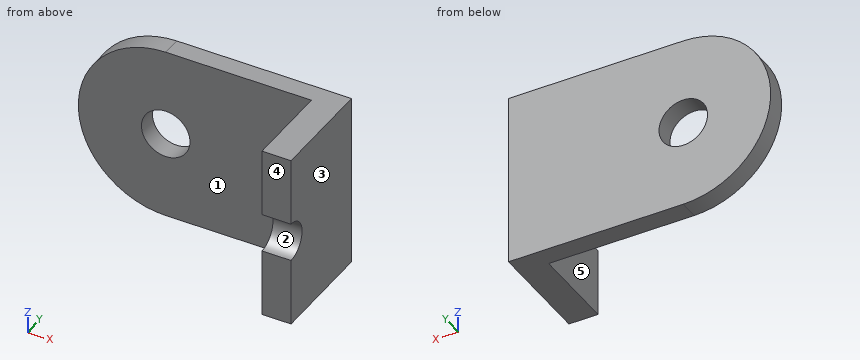
from build123d import *

# Parameters (mm, degrees)
SKETCH1_R           = 2.5
BOSS_EXTRUDE1_DEPTH = 2
BOSS_EXTRUDE2_DEPTH = 3


with BuildPart() as part:
    # Sketch1 → Boss-Extrude1 (new body)
    with BuildSketch(Plane(origin=(0, 0, 0), x_dir=(1, 0, 0), z_dir=(0, 1, 0))):
        with BuildLine():
            Line((0, 9), (18, 9))
            Line((18, 9), (18, -9))
            Line((18, -9), (0, -9))
            ThreePointArc((0, -9), (-9, 0), (0, 9))
        make_face()
        with Locations(Location((0, 0, 0), (0, 0, 270))):
            Circle(SKETCH1_R, mode=Mode.SUBTRACT)
    extrude(amount=BOSS_EXTRUDE1_DEPTH)

    # Sketch2 → Boss-Extrude2 (add)
    with BuildSketch(Plane(origin=(18, 0, 0), x_dir=(0, 0, -1), z_dir=(1, 0, 0))):
        with BuildLine():
            Line((9, 0), (-9, 0))
            Line((-9, 0), (-9, -9))
            Line((-9, -9), (-2, -9))
            ThreePointArc((-2, -9), (0, -7), (2, -9))
            Line((2, -9), (9, -9))
            Line((9, -9), (9, 0))
        make_face()
    extrude(amount=-BOSS_EXTRUDE2_DEPTH)


solid = part.part
Design review of the part built by this model. Coordinates are the model's own, in mm. Face numbers are marked on the shaded views. A direction names the side the tool comes from. Coordinates: 2 decimals unless noted, no trailing zeros. Loops run counter-clockwise (first coordinate to the right, second up) from the corner with the lowest first, then second, coordinate; pieces in that order, holes last. Notation, with made-up numbers: (25, 58) -> (34, 58) arc R7 ccw to (34, 70) -> close; hole circle Ø2 at (37.5, -8.75). An arc over 180 degrees is marked (long way). Use a Markdown table: item, result. Add a question column.
Item 1: Machinability: for the marked faces 1 and 2, which of the approach directions +Z, -Z, +X, -X, +Y, -Y give a long, thin tool a straight path to every point of the face, cutting with its end or side? Answer none if there is none.
Item 2: Clearance check with a flat-ended pin moving along its axis: P1, Ø5.5, axis at x = -1.5, z = -4.5, coming from the -Y side. State where the tip first meets the part, or that it passes through.
Item 3: We need section A-A, the plane z = 0. Write out the cut boundary in (x, y), and give its area (3 significant figures).
Item 4: We need section C-C, the plane x = 16. Write out the cut boundary in (y, z).
Item 5: Wall thickness on L1, parallel to X at y = 1.55, z = 0; L2, parallel to X at y = -0.75, z = 3.25; L3, parallel to Y at x = 9.25, z = 5.5: over which ranges is each line inside the solid? List them lowest first. Write a range as from..to.
Item 6: The part is to be moulded in two halves that separate along X. For the marked faces 3, 4 and 5, say which applies: +X half, -X half, draft (parallel to the pull), parting line (faces both ways), or undercut.
Item 7: We need section D-D, the plane z = -3.75. Write out the cut boundary in (x, y), and give its area (3 significant figures).
Item 8: We need section B-B, the plane y = -7.5. Write out the cut boundary in (x, z), and give its area (3 significant figures).
Numbers:
| question | item | result |
|---|---|---|
| 1 | face 1 | +Z, -Z, -X, -Y |
| 1 | face 2 | +X, -X, -Y |
| 2 | P1 | stops at y = 0 |
| 3 | outline | (-9, 0) -> (-2.5, 0) -> (-2.5, 2) -> (-9, 2) -> close; (2.5, 0) -> (15, 0) -> (15, -7) -> (18, -7) -> (18, 2) -> (2.5, 2) -> close |
| 3 | area | 65.0 mm^2 |
| 4 | outline | (-9, -9) -> (2, -9) -> (2, 9) -> (-9, 9) -> (-9, 2) arc R2 cw to (-9, -2) -> close |
| 5 | L1 | x = -9..-2.5, 2.5..18 |
| 5 | L2 | x = 15..18 |
| 5 | L3 | y = 0..2 |
| 6 | face 3 | +X half |
| 6 | face 4 | draft |
| 6 | face 5 | -X half |
| 7 | outline | (-8.18, 0) -> (15, 0) -> (15, -9) -> (18, -9) -> (18, 2) -> (-8.18, 2) -> close |
| 7 | area | 79.4 mm^2 |
| 8 | outline | (15, -9) -> (18, -9) -> (18, -1.32) -> (15, -1.32) -> close; (15, 1.32) -> (18, 1.32) -> (18, 9) -> (15, 9) -> close |
| 8 | area | 46.1 mm^2 |
